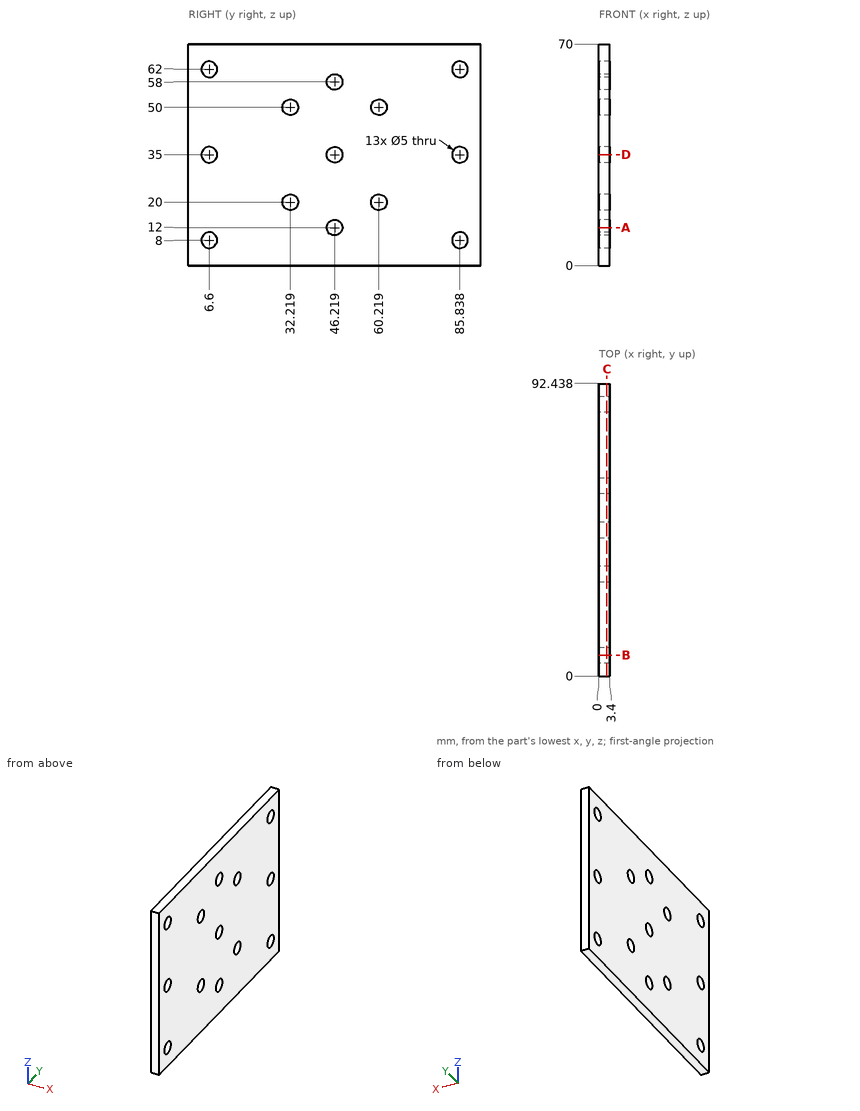
Design review of the part shown in the three views and the two pictorial views. Dimensions are in mm from the part's minimum x, y and z. Round coordinates to 2 decimals unless told otherwise and drop trailing zeros. Loops run counter-clockwise (first coordinate to the right, second up) from the corner with the lowest first, then second, coordinate; pieces in that order, holes last. Notation, with made-up numbers: (77.5, 80) - (101.5, 80) arc R24 cw to (101.5, 91) - close; hole circle Ø9 at (82, 52.5). An arc over 180 degrees is marked (long way). One line per item, written item: value. Start each with the question number.
Item 1: Take a section at D-D (z = 35). Give the boundary of the cut face in (x, y).
Item 2: Take a section at C-C (x = 2.5). State how many separate pieces and enclosed holes the cut face has.
Item 3: Take a section at A-A (z = 12). Give the boundary of the cut face in (x, y).
Item 4: Clearance check with flat-ended pins moving along their axes: pin 1 Ø6.5 at (y, z) = (32.22, 50) entering from +X; pin 2 Ø3 at (y, z) = (60.22, 20) entering from +X. State where each tip first meets the part, or that it passes through.
Item 5: For L1, parallel to Z at x = 1.45, y = 5.5 (1 decimal); L2, parallel to Y at x = 0.45, z = 20.5; L3, parallel to Z at x = 0.7, y = 84 (1 decimal), list the stretches that pass through material, from the lowest coordinate up.
Item 6: Take a section at B-B (y = 6.6). Give the boundary of the cut face in (x, z), plus the area to 3 significant figures.
Answer below:
1. outline: (0, 0) - (3.4, 0) - (3.4, 4.1) - (0, 4.1) - close; (0, 9.1) - (3.4, 9.1) - (3.4, 43.72) - (0, 43.72) - close; (0, 48.72) - (3.4, 48.72) - (3.4, 83.34) - (0, 83.34) - close; (0, 88.34) - (3.4, 88.34) - (3.4, 92.44) - (0, 92.44) - close
2. separate pieces: 1
2. enclosed holes: 13
3. outline: (0, 0) - (3.4, 0) - (3.4, 43.72) - (0, 43.72) - close; (0, 48.72) - (3.4, 48.72) - (3.4, 92.44) - (0, 92.44) - close
4. pin 1: stops at x = 3.4
4. pin 2: passes through
5. L1: z = 0 to 5.8, 10.2 to 32.8, 37.2 to 59.8, 64.2 to 70
5. L2: y = 0 to 29.77, 34.67 to 57.77, 62.67 to 92.44
5. L3: z = 0 to 6.3, 9.7 to 33.3, 36.7 to 60.3, 63.7 to 70
6. outline: (0, 0) - (3.4, 0) - (3.4, 5.5) - (0, 5.5) - close; (0, 10.5) - (3.4, 10.5) - (3.4, 32.5) - (0, 32.5) - close; (0, 37.5) - (3.4, 37.5) - (3.4, 59.5) - (0, 59.5) - close; (0, 64.5) - (3.4, 64.5) - (3.4, 70) - (0, 70) - close
6. area: 187 mm2
